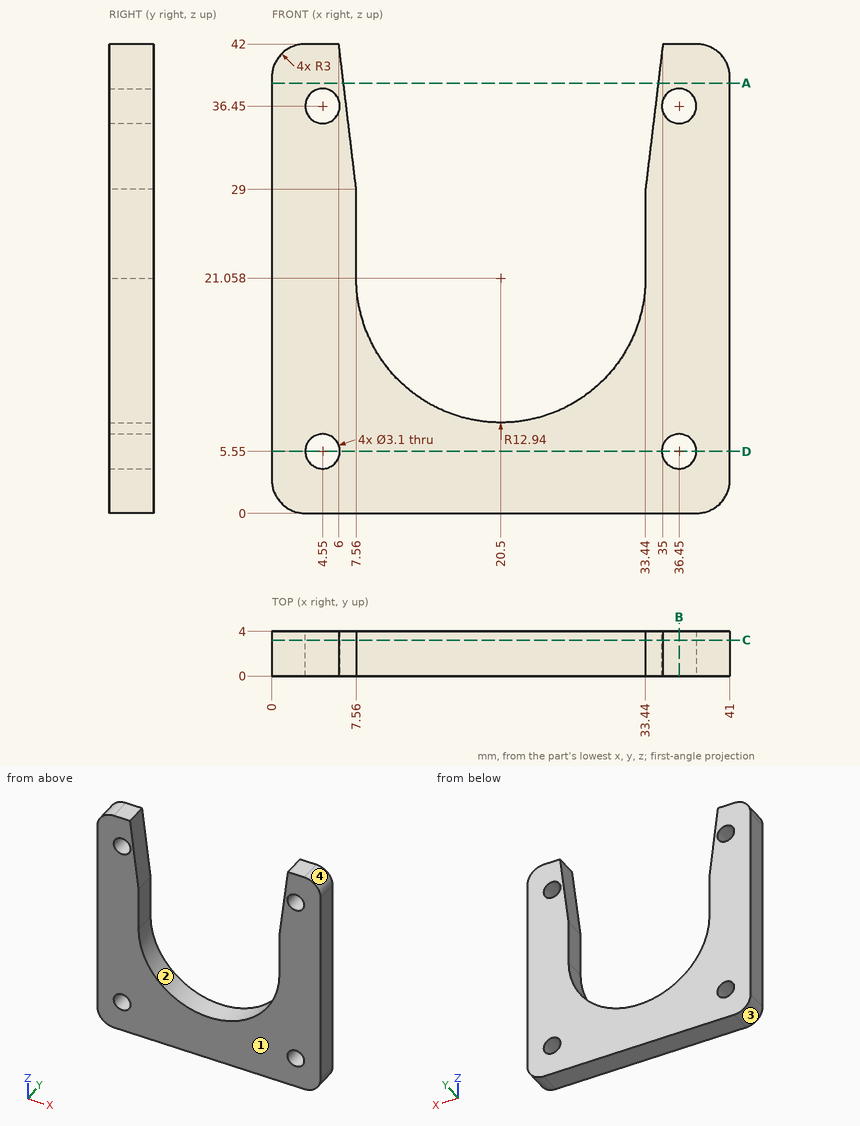
Could you check a few things on this drawing? It's one solid part, dimensions in mm from its lowest x, y, z. Give positions to 0.01 mm unless a question says otherwise; leave off trailing zeros. Write each loop counter-clockwise with the first axis right and the second up, starting at its lowest first coordinate (ties: lowest second). Pieces come first, ordered by that corner, then holes.
(1) If I drill on L1, parallel to Z at x = 36.45, y = 2.4; L2, parallel to X at y = 1.2, z = 36.45; L3, parallel to X at y = 3.05, z = 6.5 (1 decimal), over which ranges is the centre line in solid material (lowest first)?
Output values:
L1: z = 0 to 4, 7.1 to 34.9, 38 to 42
L2: x = 0 to 3, 6.1 to 6.67, 34.33 to 34.9, 38 to 41
L3: x = 0 to 3.3, 5.8 to 35.2, 37.7 to 41
(2) Imagine slicing it at C-C, the plane y = 3.2. Write out the boundary of the cut face in (x, z).
Output values:
outline: (0, 3) arc R3 ccw to (3, 0) - (38, 0) arc R3 ccw to (41, 3) - (41, 39) arc R3 ccw to (38, 42) - (35, 42) - (33.44, 29) - (33.44, 21) arc R12.94 cw to (7.56, 21) - (7.56, 29) - (6, 42) - (3, 42) arc R3 ccw to (0, 39) - close; hole circle Ø3.1 at (4.55, 5.55); hole circle Ø3.1 at (4.55, 36.45); hole circle Ø3.1 at (36.45, 5.55); hole circle Ø3.1 at (36.45, 36.45)
(3) Thinking about a two-plate mould opening in X: for the marked faces 1, 2, 3 and 4, which applies, pulls with the +X half, pulls with the -X half, needs draft (parallel to the pull), parting line crosses it, or undercut?
Output values:
face 1: needs draft
face 2: undercut
face 3: pulls with the -X half
face 4: pulls with the +X half
(4) Imagine slicing it at B-B, the plane x = 36.45. Write out the boundary of the cut face in (y, z), and give its area (3 significant figures).
Output values:
outline: (0, 0) - (4, 0) - (4, 4) - (0, 4) - close; (0, 7.1) - (4, 7.1) - (4, 34.9) - (0, 34.9) - close; (0, 38) - (4, 38) - (4, 42) - (0, 42) - close
area: 143 mm2
(5) Imagine slicing it at D-D, the plane z = 5.55. Write out the boundary of the cut face in (x, y).
Output values:
outline: (0, 0) - (3, 0) - (3, 4) - (0, 4) - close; (6.1, 0) - (34.9, 0) - (34.9, 4) - (6.1, 4) - close; (38, 0) - (41, 0) - (41, 4) - (38, 4) - close
(6) Imagine slicing it at A-A, the plane z = 38.5. Write out the boundary of the cut face in (x, y).
Output values:
outline: (0, 0) - (6.42, 0) - (6.42, 4) - (0, 4) - close; (34.58, 0) - (41, 0) - (41, 4) - (34.58, 4) - close
